from build123d import *

# Parameters (mm, degrees)
SKETCH1_W               = 3
SKETCH1_H               = 260
BOSS_EXTRUDE1_DEPTH     = 3
SKETCH2_W               = 3
SKETCH2_H               = 260
BOSS_EXTRUDE2_DEPTH     = 20.3
CUT_EXTRUDE1_DEPTH      = 22.3
CUT_EXTRUDE1_DEPTH_BACK = 20.3
SKETCH3_R               = 4.5
SKETCH5_W               = 23.3
SKETCH5_H               = 260
BOSS_EXTRUDE3_DEPTH     = 3
SKETCH6_W               = 3
SKETCH6_H               = 260
BOSS_EXTRUDE4_DEPTH     = 23.3
SKETCH8_W               = 3
SKETCH8_H               = 260
BOSS_EXTRUDE5_DEPTH     = 20.3
SKETCH11_W              = 144.5
SKETCH11_H              = 23.3
BOSS_EXTRUDE6_DEPTH     = 3
SKETCH12_W              = 138.5
SKETCH12_H              = 3
BOSS_EXTRUDE7_DEPTH     = 17
SKETCH10_R              = 6.5
CUT_EXTRUDE3_DEPTH      = 156
CUT_EXTRUDE4_START      = -10
SKETCH7_R               = 4.5
CUT_EXTRUDE4_DEPTH      = 10


with BuildPart() as part:
    # Sketch1 → Boss-Extrude1 (new body)
    with BuildSketch(Plane(origin=(0, 0, 0), x_dir=(0, 0, -1), z_dir=(1, 0, 0))):
        Rectangle(SKETCH1_W, SKETCH1_H)
    extrude(amount=BOSS_EXTRUDE1_DEPTH)

    # Sketch2 → Boss-Extrude2 (add)
    with BuildSketch(Plane(origin=(3, 0, 0), x_dir=(0, 0, -1), z_dir=(1, 0, 0))):
        Rectangle(SKETCH2_W, SKETCH2_H)
    extrude(amount=BOSS_EXTRUDE2_DEPTH)

    # Sketch3 → Cut-Extrude1 (cut, two sides: drawn at the far end of the back side and taken through both)
    with BuildSketch(Plane.XY.offset(1.5).offset(-CUT_EXTRUDE1_DEPTH_BACK)):
        with Locations(Location((15.5, 104.6, 0), (0, 0, 90))):
            Circle(SKETCH3_R)
    extrude(amount=CUT_EXTRUDE1_DEPTH + CUT_EXTRUDE1_DEPTH_BACK, mode=Mode.SUBTRACT)

    # Sketch8 → Boss-Extrude5 (add)
    with BuildSketch(Plane.XY.offset(1.5)):
        with Locations((1.5, 0)):
            Rectangle(SKETCH8_W, SKETCH8_H)
    extrude(amount=BOSS_EXTRUDE5_DEPTH)



with BuildPart() as body_2:
    # Sketch5 → Boss-Extrude3 (new body)
    with BuildSketch(Plane.XY.offset(140)):
        with Locations((11.65, 0)):
            Rectangle(SKETCH5_W, SKETCH5_H)
    extrude(amount=BOSS_EXTRUDE3_DEPTH)

    # Sketch6 → Boss-Extrude4 (add)
    with BuildSketch(Plane.XY.offset(143)):
        with Locations((1.5, 0)):
            Rectangle(SKETCH6_W, SKETCH6_H)
    extrude(amount=-BOSS_EXTRUDE4_DEPTH)


with BuildPart() as part_1:
    add(part.part)

    add(body_2.part)  # Boss-Extrude6 merges body 2
    # Sketch11 → Boss-Extrude6 (add)
    with BuildSketch(Plane(origin=(3, 0, 0), x_dir=(0, 0, -1), z_dir=(1, 0, 0))):
        with Locations((-70.75, -118.35)):
            Rectangle(SKETCH11_W, SKETCH11_H)
    extrude(amount=BOSS_EXTRUDE6_DEPTH)

    # Sketch12 → Boss-Extrude7 (add)
    with BuildSketch(Plane(origin=(6, 0, 0), x_dir=(0, 0, -1), z_dir=(1, 0, 0))):
        with Locations((-70.75, -128.5)):
            Rectangle(SKETCH12_W, SKETCH12_H)
    extrude(amount=BOSS_EXTRUDE7_DEPTH)

    # Sketch10 → Cut-Extrude3 (cut)
    with BuildSketch(Plane(origin=(0, 0, -1.5), x_dir=(-1, 0, 0), z_dir=(0, 0, -1))):
        with Locations(Location((-13, -79.4, 0), (0, 0, 90))):
            Circle(SKETCH10_R)
    extrude(amount=-CUT_EXTRUDE3_DEPTH, mode=Mode.SUBTRACT)

    # Sketch7 → Cut-Extrude4 (cut)
    with BuildSketch(Plane(origin=(0, 0, 140), x_dir=(-1, 0, 0), z_dir=(0, 0, -1)).offset(CUT_EXTRUDE4_START)):
        with Locations(Location((-15.5, 104.6, 0), (0, 0, 90))):
            Circle(SKETCH7_R)
    extrude(amount=CUT_EXTRUDE4_DEPTH, mode=Mode.SUBTRACT)


solid = part_1.part
Input: part model. Units: mm. Frame: model coordinates. A direction names the side the tool comes from. Round coordinates to 2 decimals unless told otherwise and drop trailing zeros. Loops run counter-clockwise (first coordinate to the right, second up) from the corner with the lowest first, then second, coordinate; pieces in that order, holes last. Notation, with made-up numbers: (5.25, 78.25) -> (34.25, 78.25) arc R21 ccw to (34.25, 105.25) -> close; hole circle Ø9 at (-3.5, 41.25). An arc over 180 degrees is marked (long way). Answer as a JSON object with one key per item and string values. Group by question number.
1) Draft query along Z for faces 1 (the flat face through (13, 2, 140)), 2 (the flat face through (11, -2, -1.5)), 3 (the flat face through (7, 130, 141)). Return one class per face: +Z half, -Z half, draft (parallel to the pull), parting line (faces both ways), or undercut.
2) Section query B-B on y = 104.6. Output: boundary loops of the cut face in (x, z), plus the area to 3 significant figures.
3) Pin query (flat end, axial travel): pin 1 (10.5 mm diameter, centred on x = 13, y = -79.4, fed in from +Z); pin 2 (5 mm diameter, centred on x = 19, z = 98.5, fed in from +Y); pin 3 (10 mm diameter, centred on y = -112.5, z = 61.5, fed in from +X); pin 4 (3.5 mm diameter, centred on y = -128.5, z = 65, fed in from +X). Return the tip coordinate at first contact, or that it passes through.
4) Section query D-D on z = 86. Output: boundary loops of the cut face in (x, y), plus the area to 3 significant figures.
5) Section query A-A on y = 47. Output: boundary loops of the cut face in (x, z), plus the area to 3 significant figures.
6) Reachability of faces 4 (the cylindrical face through (14.148, 108.892, -0.021)), 5 (the flat face through (3, -118, 71)), 6 (the flat face through (13, -2, 1.5)) from +Z, -Z, +X, -X, +Y, -Y: full face, straight path, thin tool, end or side. Return the list, or none.
7) Section query C-C on z = 126.5. Output: boundary loops of the cut face in (x, y), plus the area to 3 significant figures.
8) Ray query, L1, parallel to Z at x = 8.75, y = 43; L2, parallel to Y at x = 15.5, z = 140.75; L3, parallel to Z at x = 2, y = 72. Return the intervals inside material, ascending.
Reply:
{
 "1": {"face 1": "undercut", "face 2": "-Z half", "face 3": "draft"},
 "2": {"outline": "(0, -1.5) -> (11, -1.5) -> (11, 1.5) -> (3, 1.5) -> (3, 21.8) -> (0, 21.8) -> close; (0, 119.7) -> (3, 119.7) -> (3, 140) -> (11, 140) -> (11, 143) -> (0, 143) -> close; (20, -1.5) -> (23.3, -1.5) -> (23.3, 1.5) -> (20, 1.5) -> close; (20, 140) -> (23.3, 140) -> (23.3, 143) -> (20, 143) -> close", "area": "208 mm2"},
 "3": {"pin 1": "passes through", "pin 2": "stops at y = -127", "pin 3": "stops at x = 6", "pin 4": "stops at x = 23"},
 "4": {"outline": "(3, -130) -> (23, -130) -> (23, -127) -> (6, -127) -> (6, -106.7) -> (3, -106.7) -> close", "area": "121 mm2"},
 "5": {"outline": "(0, -1.5) -> (23.3, -1.5) -> (23.3, 1.5) -> (3, 1.5) -> (3, 21.8) -> (0, 21.8) -> close; (0, 119.7) -> (3, 119.7) -> (3, 140) -> (23.3, 140) -> (23.3, 143) -> (0, 143) -> close", "area": "262 mm2"},
 "6": {"face 4": "+Z, -Z", "face 5": "-X, +Y, -Y", "face 6": "+X, +Y"},
 "7": {"outline": "(0, -130) -> (23, -130) -> (23, -127) -> (6, -127) -> (6, -106.7) -> (3, -106.7) -> (3, 130) -> (0, 130) -> close", "area": "901 mm2"},
 "8": {"L1": "z = -1.5 to 1.5, 140 to 143", "L2": "y = -130 to -85.4, -73.4 to 100.1, 109.1 to 130", "L3": "z = -1.5 to 21.8, 119.7 to 143"}
}
